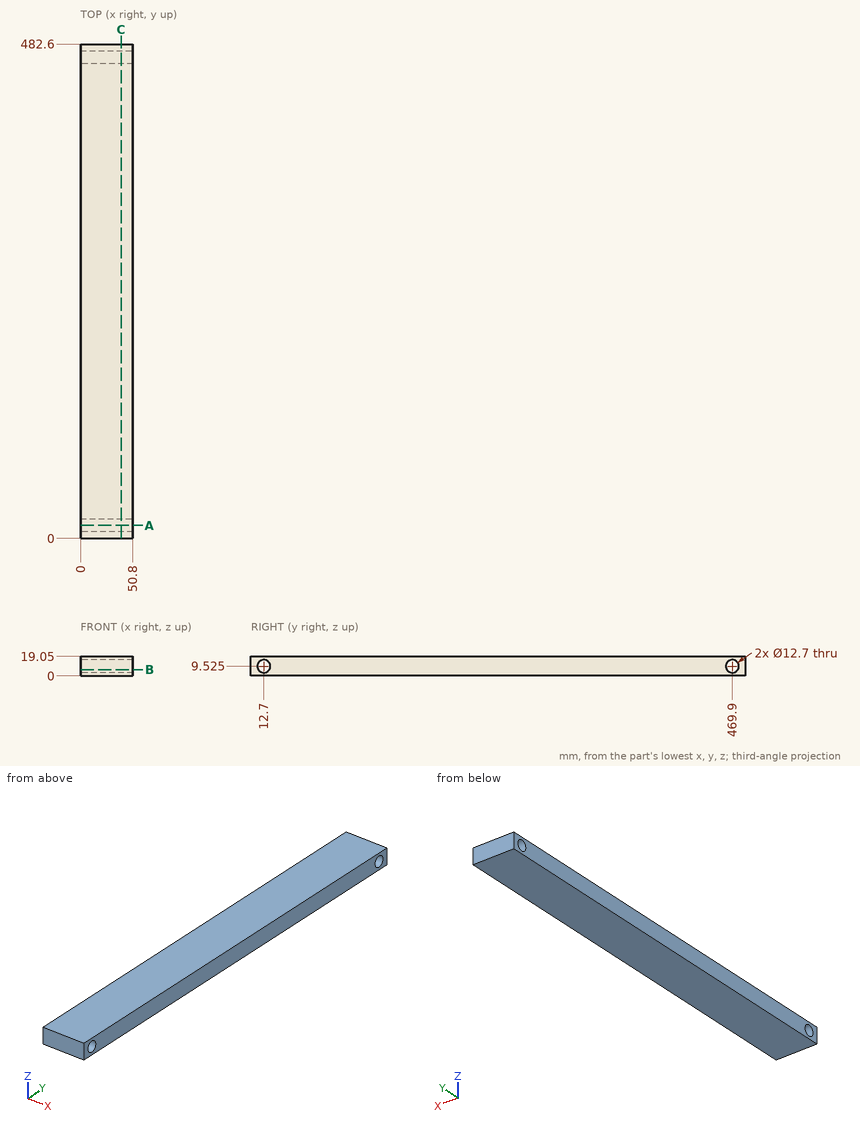
Answer from the drawing. Dimensions are ordinates in mm from the lowest x, y and z of the part. Round coordinates to 2 decimals unless told otherwise and drop trailing zeros. Write each loop counter-clockwise with the first axis right and the second up, starting at its lowest first coordinate (ties: lowest second). Pieces come first, ordered by that corner, then holes.
1. The part is cut by section B-B, the plane z = 6.25. Determine the outline of the cut face in (x, y).
2. Given pin 1 Ø3 at (x, z) = (33, 14) entering from -Y, flat-ended and moving along its own axis, determine where the tip first touches the part or whether it passes through.
3. Straight lines are drawn through the part: L1, parallel to Y at x = 15, z = 9.5; L2, parallel to Z at x = 14, y = 469.9 (3 decimals); L3, parallel to Y at x = 10.5, z = 11.5. For each, find the intervals that lie inside material, in ascending order.
4. The part is cut by section C-C, the plane x = 39.5. Determine the outline of the cut face in (y, z) (3 decimals).
5. The part is cut by section A-A, the plane y = 12.7. Determine the outline of the cut face in (x, z) (3 decimals), then the cut area to 3 significant figures.
Values:
1. outline: (0, 0) - (50.8, 0) - (50.8, 7.26) - (0, 7.26) - close; (0, 18.14) - (50.8, 18.14) - (50.8, 464.46) - (0, 464.46) - close; (0, 475.34) - (50.8, 475.34) - (50.8, 482.6) - (0, 482.6) - close
2. pin 1: stops at y = 0
3. L1: y = 0 to 6.35, 19.05 to 463.55, 476.25 to 482.6
3. L2: z = 0 to 3.175, 15.875 to 19.05
3. L3: y = 0 to 6.66, 18.74 to 463.86, 475.94 to 482.6
4. outline: (0, 0) - (482.6, 0) - (482.6, 19.05) - (0, 19.05) - close; hole circle Ø12.7 at (12.7, 9.525); hole circle Ø12.7 at (469.9, 9.525)
5. outline: (0, 0) - (50.8, 0) - (50.8, 3.175) - (0, 3.175) - close; (0, 15.875) - (50.8, 15.875) - (50.8, 19.05) - (0, 19.05) - close
5. area: 323 mm2
